Verification items for the finished model (mm, model axes). A direction names the side the tool comes from. Give positions to 0.01 mm unless a question says otherwise; leave off trailing zeros. Loops run counter-clockwise (first coordinate to the right, second up) from the corner with the lowest first, then second, coordinate; pieces in that order, holes last. Notation, with made-up numbers: (-23, 64) - (34, 64) arc R24 cw to (34, 98) - close; hole circle Ø4 at (87, 43.25). An arc over 180 degrees is marked (long way). One line per item, written item: value. Start each with the question number.
1. Mould release check, pull along Y, two halves, no side actions. Record for faces 6 (the flat face through (2, 34, 61)), 7 (the flat face through (0, 17, 61)), 8 (the cylindrical face through (23.8, 16.9, 57.5)): pulls with the +Y half, pulls with the -Y half, needs draft (parallel to the pull), parting line crosses it, or undercut.
2. Sectioned sample at C-C (y = 28.5). Record the cut outline in (x, z), plus the area to 3 significant figures.
3. Sectioned sample at A-A (x = 6.25). Record the cut outline in (y, z).
4. Sectioned sample at B-B (z = 69). Record the cut outline in (x, y), plus the area to 3 significant figures.
5. Access from +Z, -Z, +X, -X, +Y, -Y to the whole of each face (thin tool, end or side, straight path). Record for faces 1 (the flat face through (23, 19, 63)), 2 (the flat face through (22.76, 17.5, 63.8)), 3 (the flat face through (2, 17, 0)), 4 (the flat face through (19, 21, 62)), 5 (the flat face through (12.5, 23, 63)).
6. Gauge pin test, flat ends, axial feed: pin 1 (7 mm diameter, centred on x = 24, z = 64.1, fed in from -Y); pin 2 (6 mm diameter, centred on y = 19, z = 82, fed in from +X); pin 3 (4 mm diameter, centred on x = 23.5, z = 64, fed in from +Y); pin 4 (4 mm diameter, centred on x = 7.5, y = 6.5, fed in from +Z). Record the tip position at first contact, or that the pin passes through.
7. Scan lines: L1, parallel to X at y = 14.05, z = 64.1; L2, parallel to X at y = 18.05, z = 64.1; L3, parallel to Z at x = 24, y = 18.75. Record each from-to range of solid material in increasing order. Write a range as [from, to].
8. Sectioned sample at D-D (x = 14.5). Record the cut outline in (y, z), plus the area to 3 significant figures.
from build123d import *

# Parameters (mm, degrees)
SKETCH1_W                                     = 120
SKETCH1_H                                     = 34
BOSS_EXTRUDE1_DEPTH                           = 5
BOSS_EXTRUDE2_DEPTH                           = 7.5
SKETCH3_R                                     = 6
BOSS_EXTRUDE3_DEPTH                           = 16
CUT_EXTRUDE1_DEPTH                            = 9.5
SKETCH5_W                                     = 0.5
SKETCH5_H                                     = 12
CUT_EXTRUDE2_DEPTH                            = 8.5
CBORE_START                                   = 19
CBORE_FOR_M2_HEX_SOCKET_HEAD_CAP_SCREW1_DEPTH = 3.691221609
CBORE_START_2                                 = 17.5
CBORE_FOR_M2_HEX_SOCKET_HEAD_CAP_SCR_3_O_R    = 1.1
CBORE_FOR_M2_HEX_SOCKET_HEAD_CAP_SCR_3_DEPTH  = 1.5
M2_TAPPED_HOLE1_D                             = 1.6
FILLET1_R                                     = 0.2


# Read off the part's stored shape, not the designer's step: CBORE for M2 Hex Socket Head Cap Screw1
with BuildPart() as part:
    # Sketch1 → Boss-Extrude1 (new body)
    with BuildSketch(Plane(origin=(0, 0, 0), x_dir=(0, 0, -1), z_dir=(1, 0, 0))):
        with Locations((-60, 17)):
            Rectangle(SKETCH1_W, SKETCH1_H)
    extrude(amount=BOSS_EXTRUDE1_DEPTH)

    # Sketch2 → Boss-Extrude2 (add)
    with BuildSketch(Plane(origin=(5, 0, 0), x_dir=(0, 0, -1), z_dir=(1, 0, 0))):
        with BuildLine():
            ThreePointArc((-52.5, 17), (-54.696699141, 22.303300859), (-60, 24.5))
            Line((-60, 24.5), (-60, 9.5))
            ThreePointArc((-60, 9.5), (-54.696699141, 11.696699141), (-52.5, 17))
        make_face()
        with BuildLine():
            Line((-60, 9.5), (-60, 24.5))
            ThreePointArc((-60, 24.5), (-67.5, 17), (-60, 9.5))
        make_face()
    extrude(amount=BOSS_EXTRUDE2_DEPTH)

    # Sketch3 → Boss-Extrude3 (add)
    with BuildSketch(Plane(origin=(12.5, 0, 0), x_dir=(0, 0, -1), z_dir=(1, 0, 0))):
        with Locations((-60, 17)):
            Circle(SKETCH3_R)
    extrude(amount=BOSS_EXTRUDE3_DEPTH)

    # Sketch4 → Cut-Extrude1 (cut)
    with BuildSketch(Plane(origin=(28.5, 0, 0), x_dir=(0, 0, -1), z_dir=(1, 0, 0))):
        with BuildLine():
            Line((-62.449489743, 17.5), (-67.449489743, 17.5))
            Line((-67.449489743, 17.5), (-67.449489743, 16.5))
            Line((-67.449489743, 16.5), (-62.449489743, 16.5))
            ThreePointArc((-62.449489743, 16.5), (-57.5, 17), (-62.449489743, 17.5))
        make_face()
    extrude(amount=-CUT_EXTRUDE1_DEPTH, mode=Mode.SUBTRACT)

    # Sketch5 → Cut-Extrude2 (cut)
    with BuildSketch(Plane.XY.offset(66)):
        with Locations((18.75, 17)):
            Rectangle(SKETCH5_W, SKETCH5_H)
    extrude(amount=-CUT_EXTRUDE2_DEPTH, mode=Mode.SUBTRACT)

    # CBORE for M2 Hex Socket Head Cap Scr 2 → CBORE for M2 Hex Socket Head Cap Screw1 (cut)
    with BuildSketch(Plane(origin=(0, 0, 0), x_dir=(1, 0, 0), z_dir=(0, 1, 0)).offset(CBORE_START)):
        with BuildLine():
            Line((24.209160843, -67), (25.554414631, -65.656854249))
            ThreePointArc((25.554414631, -65.656854249), (24, -61.9), (22.445585369, -65.656854249))
            Line((22.445585369, -65.656854249), (23.790839157, -67))
            Line((23.790839157, -67), (24.209160843, -67))
        make_face()
    extrude(amount=CBORE_FOR_M2_HEX_SOCKET_HEAD_CAP_SCREW1_DEPTH, mode=Mode.SUBTRACT)

    # CBORE for M2 Hex Socket Head Cap Scr 3 o → CBORE for M2 Hex Socket Head Cap Scr 3 (cut)
    with BuildSketch(Plane(origin=(0, 0, 0), x_dir=(1, 0, 0), z_dir=(0, 1, 0)).offset(CBORE_START_2)):
        with Locations((24, -64.1)):
            Circle(CBORE_FOR_M2_HEX_SOCKET_HEAD_CAP_SCR_3_O_R)
    extrude(amount=CBORE_FOR_M2_HEX_SOCKET_HEAD_CAP_SCR_3_DEPTH, mode=Mode.SUBTRACT)

    # M2 Tapped Hole1 (through all)
    with Locations(Plane(origin=(0, 16.5, 0), x_dir=(1, 0, 0), z_dir=(0, 1, 0))):
        with Locations((24, -64.1)):
            Hole(M2_TAPPED_HOLE1_D / 2)

    # Fillet1
    fillet1_edges = [part.edges().sort_by_distance(p)[0] for p in [
        (5, 24.5, 60),
        (12.5, 17, 66),
    ]]
    fillet(fillet1_edges, radius=FILLET1_R)


solid = part.part
Results are:
1. face 6: pulls with the +Y half
1. face 7: needs draft
1. face 8: undercut
2. outline: (0, 0) - (5, 0) - (5, 120) - (0, 120) - close
2. area: 600 mm^2
3. outline: circle Ø15 at (17, 60)
4. outline: (0, 0) - (5, 0) - (5, 34) - (0, 34) - close
4. area: 170 mm^2
5. face 1: +Y
5. face 2: +Z, +X
5. face 3: -Z, +X, -X, +Y, -Y
5. face 4: +Z, +Y, -Y
5. face 5: +X
6. pin 1: stops at y = 11.03
6. pin 2: stops at x = 5
6. pin 3: stops at y = 22.65
6. pin 4: passes through
7. L1: x = [0, 18.5], [19, 23.2], [24.8, 28.5]
7. L2: x = [0, 18.5], [19, 22.9], [25.1, 28.5]
7. L3: z = [54.26, 58.21], [61.79, 63], [65.2, 65.74]
8. outline: circle Ø12 at (17, 60)
8. area: 113 mm^2
